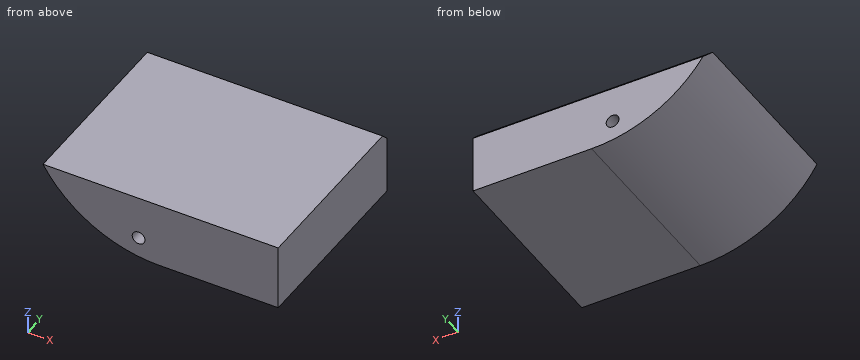
from build123d import *

# Parameters (mm, degrees)
F0_W        = 150
F0_H        = 120.4859416558
F1_DEPTH    = 42
F2_SIZE     = 5
F3_T1_DEPTH = 492.526994922
F6_R        = 4.0747978112
F7_DEPTH    = 192


# Not quite as in the source:
# - a fillet or chamfer that OpenCascade refuses, or shapes differently, is made with other operations: its cross-section is extruded or revolved along the edge and cut away or added
# - the program builds the solid bodies; features that only make, move or delete a surface that nothing else refers to are left out


with BuildPart() as f1:
    # F0 (on Top) → F1 (new body)
    with BuildSketch(Plane.XY):
        with Locations((-21.8634653855, -60.2429708279)):
            Rectangle(F0_W, F0_H)
    extrude(amount=F1_DEPTH)

    # F2
    f2_edges = [f1.edges().sort_by_distance(p)[0] for p in [
        (-21.863465, 0, 42),
    ]]
    chamfer(f2_edges, length=F2_SIZE)

    # F3: fillet of radius 86.9116882454 on 1 edges, made by hand

    # F3_s2 → F3_t1 (cut)
    with BuildSketch(Plane.XZ.offset(-186.0205266331)):
        with BuildLine():
            ThreePointArc((-22.4552547323, 0), (-65.1769758253, 11.2248591368), (-96.8634653855, 42))
            Line((-96.8634653855, 42), (-96.8634653855, 0))
            Line((-96.8634653855, 0), (-22.4552547323, 0))
        make_face()
    extrude(amount=F3_T1_DEPTH, mode=Mode.SUBTRACT)

    # F6 (on face) → F7 (cut)
    with BuildSketch(Plane.XZ.offset(120.4859416558)):
        with Locations((-35.8820706606, 14.1489794478)):
            Circle(F6_R)
    extrude(amount=-F7_DEPTH, mode=Mode.SUBTRACT)


solid = f1.part
Model file for the job. Use its own axes, mm. Give positions to 0.01 mm unless a question says otherwise; leave off trailing zeros. Order: outer loops, then holes, each group sorted by start corner. A loop starts at its lowest first (then second) coordinate and runs counter-clockwise, first axis right, second up. Notation, with made-up numbers: (57.5, 70.5) - (70.5, 70.5) arc R32 ccw to (70.5, 99.5) - close; hole circle Ø7 at (-24.5, 23.5). An arc over 180 degrees is marked (long way). Write item = value, one per line. Start each with the question number.
1. Cut at D-D, the plane x = -84. List the corners of the cut face in (y, z).
2. Cut at C-C, the plane z = 20. List the corners of the cut face in (x, y).
3. Cut at B-B, the plane x = -68.5. List the corners of the cut face in (y, z).
4. Drop flat-ended pins along their axis: P1, Ø6.5, axis at x = -35.88, z = 14.15, coming from the +Y side; P2, Ø12, axis at y = -98, z = 17, coming from the -X side. Give the stop position or say it passes through.
5. Probe line 1 along X through (y, z) = (-83, 14.5); line 2 along X through (y, z) = (-23, 17); line 3 along Z through (x, y) = (-24, -83.5). List the from-to ranges inside material, lowest first.
6. Cut at A-A, the plane y = -97.5. List the corners of the cut face in (x, z), and give its area (3 significant figures).
Taken from the geometry:
q1.outline = (-120.49, 25.54) - (0, 25.54) - (0, 37) - (-5, 42) - (-120.49, 42) - close
q2.outline = (-77.92, -120.49) - (53.14, -120.49) - (53.14, 0) - (-77.92, 0) - close
q3.outline = (-120.49, 13.2) - (0, 13.2) - (0, 37) - (-5, 42) - (-120.49, 42) - close
q4.P1 = through
q4.P2 = -81.35
q5.line_1 = -70.52 to -39.94, -31.82 to 53.14
q5.line_2 = -74.09 to -38.79, -32.97 to 53.14
q5.line_3 = 0.01 to 42
q6.outline = (-96.86, 42) arc R86.91 ccw to (-22.46, 0) - (53.14, 0) - (53.14, 42) - close; hole circle Ø8.15 at (-35.88, 14.15)
q6.area = 5,330 mm²
